Can you work these out from the model? Positions are in its coordinate system, mm. A direction names the side the tool comes from. Give positions to 0.01 mm unless a question says otherwise; leave off trailing zeros. Loops run counter-clockwise (first coordinate to the right, second up) from the corner with the lowest first, then second, coordinate; pieces in that order, holes last. Notation, with made-up numbers: (-19, 74) - (-14, 74) arc R31 ccw to (-14, 109) - close; hole circle Ø8 at (23, -10.5). An arc over 180 degrees is marked (long way). Answer in a Markdown table with one row per item.
from build123d import *

# Parameters (mm, degrees)
SKETCH1_R           = 6.5
BOSS_EXTRUDE1_DEPTH = 60
SKETCH2_R           = 3
INNER_CHAMBER_DEPTH = 52.5
SKETCH4_R           = 7.25
BOSS_EXTRUDE2_DEPTH = 6
FILLET4_R           = 0.1
FILLET5_R           = 0.25
FILLET6_R           = 0.25


with BuildPart() as part:
    # Sketch1 → Boss-Extrude1 (new body)
    with BuildSketch(Plane(origin=(0, 0, 0), x_dir=(1, 0, 0), z_dir=(0, 1, 0))):
        with Locations(Location((0, 0, 0), (0, 0, 270))):
            Circle(SKETCH1_R)
    extrude(amount=BOSS_EXTRUDE1_DEPTH)

    # Sketch2 → Inner Chamber (cut)
    with BuildSketch(Plane(origin=(0, 60, 0), x_dir=(1, 0, 0), z_dir=(0, 1, 0))):
        with Locations(Location((0, 0, 0), (0, 0, 270))):
            Circle(SKETCH2_R)
    extrude(amount=-INNER_CHAMBER_DEPTH, mode=Mode.SUBTRACT)

    # Sketch4 → Boss-Extrude2 (add)
    with BuildSketch(Plane.XZ):
        with Locations(Location((0, 0, 0), (0, 0, 270))):
            Circle(SKETCH4_R)
    extrude(amount=BOSS_EXTRUDE2_DEPTH)

    # Sketch6 → Revolve1 (revolve)
    with BuildSketch(Plane(origin=(0, 0, 0), x_dir=(0, 0, -1), z_dir=(1, 0, 0))):
        Polygon((1, -6), (6.75, -12), (7, -12), (4, -6), align=None)
    revolve(axis=Axis((0, -6, 0), (0, -1, 0)))

    # Fillet4
    fillet4_edges = [part.edges().sort_by_distance(p)[0] for p in [
        (0, -12, 7),
        (0, -12, 6.75),
    ]]
    fillet(fillet4_edges, radius=FILLET4_R)

    # Fillet5
    fillet5_edges = [part.edges().sort_by_distance(p)[0] for p in [
        (0, -6, 7.25),
    ]]
    fillet(fillet5_edges, radius=FILLET5_R)

    # Fillet6
    fillet6_edges = [part.edges().sort_by_distance(p)[0] for p in [
        (0, -6, 4),
    ]]
    fillet(fillet6_edges, radius=FILLET6_R)


solid = part.part
Q1. Imagine slicing it at C-C, the plane z = 0. Write out the boundary of the cut face in (x, y), and give its area (3 significant figures).
Checked values:
| item | result |
|---|---|
| outline | (-7.25, -5.75) arc R0.25 ccw to (-7, -6) - (-4.4, -6) arc R0.25 cw to (-4.18, -6.36) - (-6.93, -11.86) arc R0.1 ccw to (-6.84, -12) - (-6.79, -12) arc R0.1 ccw to (-6.72, -11.97) - (-1, -6) - (1, -6) - (6.72, -11.97) arc R0.1 ccw to (6.79, -12) - (6.84, -12) arc R0.1 ccw to (6.93, -11.86) - (4.18, -6.36) arc R0.25 cw to (4.4, -6) - (7, -6) arc R0.25 ccw to (7.25, -5.75) - (7.25, 0) - (6.5, 0) - (6.5, 60) - (3, 60) - (3, 7.5) - (-3, 7.5) - (-3, 60) - (-6.5, 60) - (-6.5, 0) - (-7.25, 0) - close |
| area | 572 mm² |
Q2. Imagine slicing it at D-D, the plane y = 3.5. Write out the boundary of the cut face in (x, z).
Checked values:
| item | result |
|---|---|
| outline | circle Ø13 at (0, 0) |
Q3. If we mould it in two halves opening along X, with no side actions, what happens to faces 4 (the face through (-4.21, -6.63, 0.94)), 5 (the face through (-1, 60, 3)), 6 (the face through (0.9, 34.12, 2.86))? For each: released by +X, released by -X, zero draft, split by the parting line, or undercut.
Checked values:
| item | result |
|---|---|
| face 4 | split by the parting line |
| face 5 | zero draft |
| face 6 | undercut |
Q4. For pin 1 (1.5 mm diameter, centred on x = 3, y = 43.5, fed in from +Z); pin 2 (2 mm diameter, centred on y = 36, z = 2.5, fed in from -X); pin 3 (6 mm diameter, centred on x = 0.5, y = 39, fed in from +Z), each with a flat end and sliding along its axis, tell me the tip position at first contact or that it passes through.
Checked values:
| item | result |
|---|---|
| pin 1 | stops at z = 6.1 |
| pin 2 | stops at x = -6.32 |
| pin 3 | stops at z = 6.5 |
Q5. If I drill on line 1 (X direction, y = 29, z = 0); line 2 (Z direction, x = 1, y = 18.5); line 3 (X direction, y = 30, z = 1.75), over which ranges is the centre line in solid material (lowest first)? Write a range as [from, to].
Checked values:
| item | result |
|---|---|
| line 1 | x = [-6.5, -3], [3, 6.5] |
| line 2 | z = [-6.42, -2.83], [2.83, 6.42] |
| line 3 | x = [-6.26, -2.44], [2.44, 6.26] |
Q6. Imagine slicing it at B-B, the plane y = 49.5. Write out the boundary of the cut face in (x, z), and give its area (3 significant figures).
Checked values:
| item | result |
|---|---|
| outline | circle Ø13 at (0, 0); hole circle Ø6 at (0, 0) |
| area | 104 mm² |
Q7. On a 3-axis mill with a long thin cutter (end or side, diameter ignored), from which of +Z, -Z, +X, -X, +Y, -Y can I reach the whole of each face in a straight line? I mean faces 1 (the face through (0, -6, 0)), 2 (the face through (0, 7.5, 0)), 3 (the face through (-5, -6, 0)). Say none if no direction works.
Checked values:
| item | result |
|---|---|
| face 1 | -Y |
| face 2 | +Y |
| face 3 | none |
Q8. Imagine slicing it at A-A, the plane x = 0. Write out the boundary of the cut face in (y, z), and give its area (3 significant figures).
Checked values:
| item | result |
|---|---|
| outline | (-12, -6.84) arc R0.1 ccw to (-11.86, -6.93) - (-6.36, -4.18) arc R0.25 cw to (-6, -4.4) - (-6, -7) arc R0.25 ccw to (-5.75, -7.25) - (0, -7.25) - (0, -6.5) - (60, -6.5) - (60, -3) - (7.5, -3) - (7.5, 3) - (60, 3) - (60, 6.5) - (0, 6.5) - (0, 7.25) - (-5.75, 7.25) arc R0.25 ccw to (-6, 7) - (-6, 4.4) arc R0.25 cw to (-6.36, 4.18) - (-11.86, 6.93) arc R0.1 ccw to (-12, 6.84) - (-12, 6.79) arc R0.1 ccw to (-11.97, 6.72) - (-6, 1) - (-6, -1) - (-11.97, -6.72) arc R0.1 ccw to (-12, -6.79) - close |
| area | 572 mm² |
